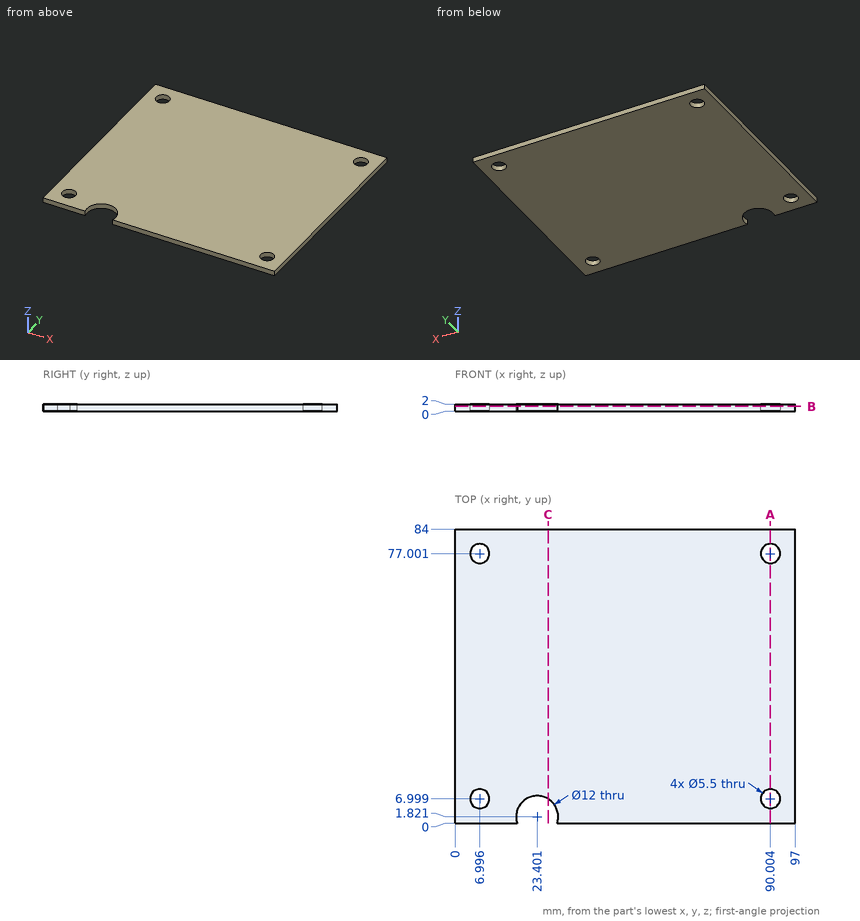
Answer from the drawing. Dimensions are ordinates in mm from the lowest x, y and z of the part. Round coordinates to 2 decimals unless told otherwise and drop trailing zeros. Order: outer loops, then holes, each group sorted by start corner. A loop starts at its lowest first (then second) coordinate and runs counter-clockwise, first axis right, second up.
1) The part is cut by section B-B on z = 1.35. Give the number of separate pieces and of enclosed holes in the cut face.
2) The part is cut by section C-C on x = 26.5. Write down the section's boundary in (y, z), plus the area to 3 significant figures.
3) Straight lines are drawn through the part: L1, parallel to Y at x = 9.5, z = 0.45 (1 decimal); L2, parallel to Y at x = 8, z = 0.65; L3, parallel to X at y = 8.5, z = 1.3. For each, find the intervals that lie inside material, in ascending order.
4) The part is cut by section A-A on x = 90. Write down the section's boundary in (y, z).
5) Flat-ended cylindrical pins translate along their axes: pin 1 (9 mm diameter, centred on x = 7, y = 7, fed in from +Z); pin 2 (7 mm diameter, centred on x = 23.4, y = 1.82, fed in from +Z). Find the tip coordinate at first contact, or state that the pin passes through.
Resolved:
1. separate pieces: 1
1. enclosed holes: 4
2. outline: (6.96, 0) - (84, 0) - (84, 2) - (6.96, 2) - close
2. area: 154 mm2
3. L1: y = 0 to 5.9, 8.1 to 75.9, 78.1 to 84
3. L2: y = 0 to 4.44, 9.56 to 74.44, 79.56 to 84
3. L3: x = 0 to 4.69, 9.3 to 87.7, 92.31 to 97
4. outline: (0, 0) - (4.25, 0) - (4.25, 2) - (0, 2) - close; (9.75, 0) - (74.25, 0) - (74.25, 2) - (9.75, 2) - close; (79.75, 0) - (84, 0) - (84, 2) - (79.75, 2) - close
5. pin 1: stops at z = 2
5. pin 2: passes through
